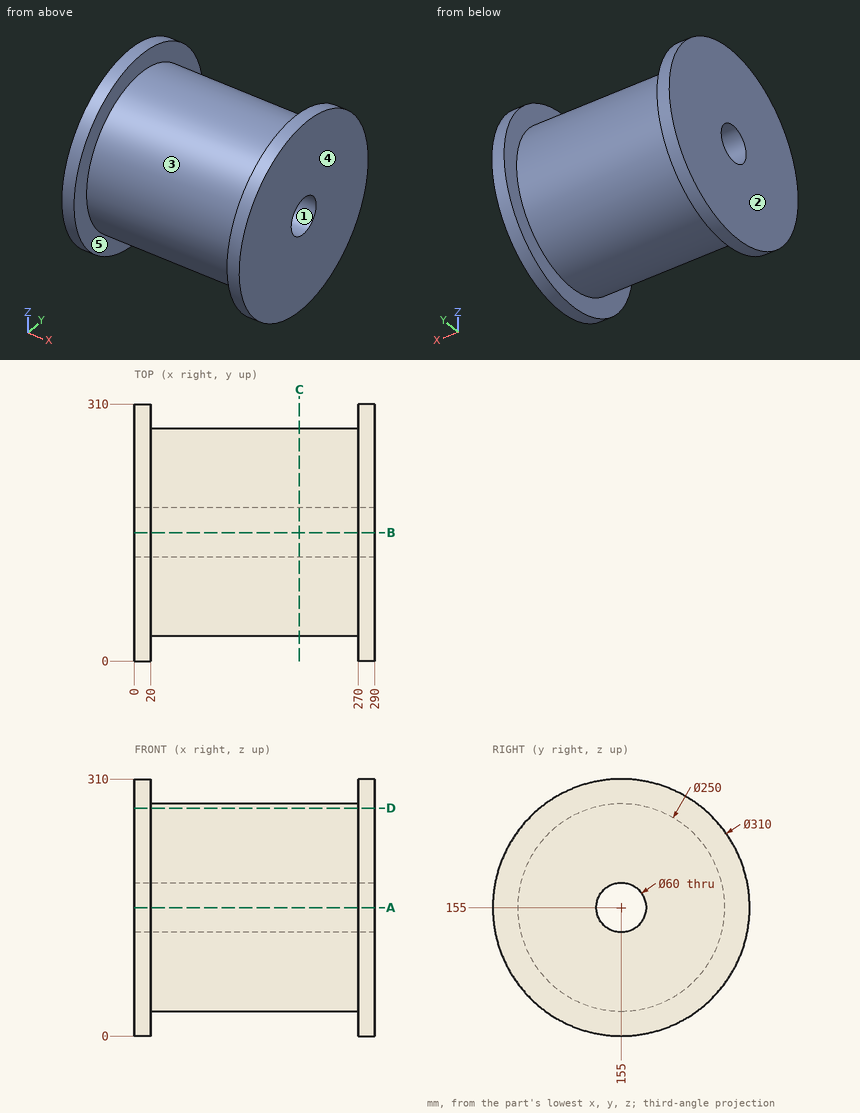
Verification items for this drawing (mm, ordinates from the low corner). A direction names the side the tool comes from. Coordinates: 2 decimals unless noted, no trailing zeros. Loops run counter-clockwise (first coordinate to the right, second up) from the corner with the lowest first, then second, coordinate; pieces in that order, holes last.
Item 1: Sectioned sample at C-C, the plane x = 199. Record the boundary of the cut face in (y, z).
Item 2: Sectioned sample at D-D, the plane z = 275. Record the boundary of the cut face in (x, y), then the cut area to 3 significant figures.
Item 3: Thickness scan on line 1 (Y direction, x = 83, z = 155); line 2 (X direction, y = 58.5, z = 58.5); line 3 (Y direction, x = 146, z = 127.5). Record the ranges inside material, lowest first.
Item 4: Release check for a two-part mould opening along Y. For the marked faces 1, 2 and 3 record: released by +Y, released by -Y, zero draft, split by the parting line, or undercut.
Item 5: Sectioned sample at A-A, the plane z = 155. Record the boundary of the cut face in (x, y), then the cut area to 3 significant figures.
Item 6: Go/stop test with flat-tipped pins: pin 1 Ø3 at (x, y) = (94.5, 202) entering from -Z; pin 2 Ø8 at (x, y) = (258, 178) entering from +Z; pin 3 Ø10 at (x, y) = (121.5, 155) entering from +Z. Record where each tip stops, or that it passes through.
Item 7: Access from +Z, -Z, +X, -X, +Y, -Y to the whole of each face (thin tool, end or side, straight path). Record for the marked faces 4 and 5.
Check result:
1. outline: circle Ø250 at (155, 155); hole circle Ø60 at (155, 155)
2. outline: (0, 56.89) - (20, 56.89) - (20, 120) - (270, 120) - (270, 56.89) - (290, 56.89) - (290, 253.11) - (270, 253.11) - (270, 190) - (20, 190) - (20, 253.11) - (0, 253.11) - close
2. area: 25,300 mm2
3. line 1: y = 30 to 125, 185 to 280
3. line 2: x = 0 to 20, 270 to 290
3. line 3: y = 33.06 to 143.01, 166.99 to 276.94
4. face 1: undercut
4. face 2: zero draft
4. face 3: split by the parting line
5. outline: (0, 0) - (20, 0) - (20, 30) - (270, 30) - (270, 0) - (290, 0) - (290, 125) - (0, 125) - close; (0, 185) - (290, 185) - (290, 310) - (270, 310) - (270, 280) - (20, 280) - (20, 310) - (0, 310) - close
5. area: 57,500 mm2
6. pin 1: stops at z = 38.58
6. pin 2: stops at z = 278.55
6. pin 3: stops at z = 280
7. face 4: +Z, -Z, +X, +Y, -Y
7. face 5: none
